Here's how the part is built. I have some questions about the finished solid (model axes, mm). A direction names the side the tool comes from. Give positions to 0.01 mm unless a question says otherwise; leave off trailing zeros. Write each loop counter-clockwise with the first axis right and the second up, starting at its lowest first coordinate (ties: lowest second). Pieces come first, ordered by that corner, then holes. Notation, with made-up numbers: (2, 65) -> (41, 65) arc R26 cw to (41, 86) -> close; hole circle Ø7 at (-10, 6.5). An arc over 180 degrees is marked (long way). Use one line per item in the form item = value.
Autodesk Inventor part; units mm, degrees
ref_plane "YZ Plane" through (0, 0, 0) normal (1, 0, 0) x (0, 1, 0)
ref_plane "XZ Plane" through (0, 0, 0) normal (0, 1, 0) x (-1, 0, 0)
ref_plane "XY Plane" through (0, 0, 0) normal (0, 0, 1) x (1, 0, 0)
sketch "Base" plane through (0, 0, 0) normal (0, 1, 0) x (-1, 0, 0)
  line L0 (92, 60.5) -> (-92, 60.5)
  line L1 (-92, 60.5) -> (-92, -60.5)
  line L2 (-92, -60.5) -> (92, -60.5)
  line L3 (92, -60.5) -> (92, 60.5)
  line L4 (92, 60.5) -> (-92, -60.5) construction
  line L5 (-92, 60.5) -> (92, -60.5) construction
  point P0 (0, 0)
  dimension "d0" = 184
  dimension "d1" = 121
extrude "Extrusão1" add sketch "Base" against normal blind 26
sketch "Esboço2" plane through (0, 0, 0) normal (0, 1, 0) x (1, 0, 0)
  line L0 (-90, -58.5) -> (90, -58.5)
  line L1 (90, -58.5) -> (90, 58.5)
  line L2 (90, 58.5) -> (-90, 58.5)
  line L3 (-90, 58.5) -> (-90, -58.5)
  line L4 (-90, -58.5) -> (90, 58.5) construction
  line L5 (90, -58.5) -> (-90, 58.5) construction
  point P0 (0, 0)
  dimension "d4" = 180
  dimension "d5" = 117
extrude "Extrusão2" cut sketch "Esboço2" against normal blind 22
sketch "Esboço3" plane through (0, -22, 0) normal (0, 1, 0) x (1, 0, 0)
  circle A0 centre (-85, -53.5) radius 2.5
  line L0 (-92, 60.5) -> (-92, -60.5)
  line L1 (-92, -60.5) -> (92, -60.5)
  circle A1 centre (-85, -53.5) radius 1.5
  line L2 (-90, -58.5) -> (-90, 58.5)
  line L3 (90, 58.5) -> (90, -58.5)
  circle A2 centre (-85, 53.5) radius 2.5
  circle A3 centre (-85, 53.5) radius 1.5
  line L4 (-90, 58.5) -> (90, 58.5)
  line L5 (90, -58.5) -> (-90, -58.5)
  circle A4 centre (85, 53.5) radius 1.5
  circle A5 centre (85, 53.5) radius 2.5
  line L6 (92, -60.5) -> (92, 60.5)
  line L7 (92, 60.5) -> (-92, 60.5)
  circle A6 centre (76.27, -28.99) radius 2.5
  circle A7 centre (76.27, -28.99) radius 1.5
  point P0 (0, 0)
  dimension "d8" = 5
  dimension "d9" = 7
  dimension "d10" = 7
  dimension "d11" = 3
  dimension "d12" = 7
  dimension "d13" = 7
  dimension "d14" = 5
  dimension "d15" = 31.51
  dimension "d16" = 15.73
  dimension "d17" = 3
extrude "Extrusão3" add sketch "Esboço3" along normal blind 4 contours A0 | A2 | A5 | A6
sketch "Esboço4" plane through (92, 0, -60.5) normal (0, 0, -1) x (-1, 0, 0)
  line L0 (92, 0) -> (64, 0)
  line L1 (64, 0) -> (64, -4)
  line L2 (64, -4) -> (92, -4)
  line L3 (92, -4) -> (92, 0)
  line L4 (92, 0) -> (64, -4) construction
  line L5 (64, 0) -> (92, -4) construction
  line L6 (184, 0) -> (184, -26)
  line L7 (0, 0) -> (184, 0)
  line L8 (184, -26) -> (0, -26)
  point P0 (92, 0)
  point P1 (78, -2)
  point P2 (64, -2)
  dimension "d20" = 120
  dimension "d21" = 28
  dimension "d22" = 0
  dimension "d24" = 4
extrude "Extrusão4" cut sketch "Esboço4" along normal blind 4 and the other way blind 2
properties part number "base_traseira_3DPrint"
Q1. I want a section at A-A, the plane z = -27. Write out the boundary of the cut face in (x, y).
Result set:
outline = (-92, -26) -> (92, -26) -> (92, 0) -> (90, 0) -> (90, -22) -> (-90, -22) -> (-90, 0) -> (-92, 0) -> close
Q2. If I drill on line 1 along Z through (x, y) = (-85, -19.6); line 2 along X through (y, z) = (-20.9, -53.5); line 3 along X through (y, z) = (-6.25, 45.5), over which ranges is the centre line in solid material (lowest first)? Write a range as from..to.
Result set:
line_1 = -60.5..-58.5, -56..-55, -52..-51, 51..52, 55..56, 58.5..60.5
line_2 = -92..-90, -87.5..-86.5, -83.5..-82.5, 82.5..83.5, 86.5..87.5, 90..92
line_3 = -92..-90, 90..92
Q3. I want a section at B-B, the plane y = -14.5. Write out the boundary of the cut face in (x, z), and give its area (3 significant figures).
Result set:
outline = (-92, -60.5) -> (92, -60.5) -> (92, 60.5) -> (-92, 60.5) -> close; hole (-90, -58.5) -> (90, -58.5) -> (90, 58.5) -> (-90, 58.5) -> close
area = 1,200 mm2
Q4. Will these pins go through, and if not, where does the flat tip stop? pin 1 Ø3.5 at (x, z) = (-85, -53.5) entering from +Y; pin 2 Ø12 at (x, z) = (-6.5, 23) entering from +Y; pin 3 Ø2 at (x, z) = (20, -59.5) entering from +Y.
Result set:
pin_1 = -18
pin_2 = -22
pin_3 = -4
Q5. If we mould it in two halves opening along Z, with no side actions, what happens to faces 1 (the face through (1, -26, 1)), 2 (the face through (1, -11, -58.5)), 3 (the face through (1, -13, -60.5))? For each: +Z half, -Z half, draft (parallel to the pull), parting line (faces both ways), or undercut.
Result set:
face_1 = draft
face_2 = undercut
face_3 = -Z half
Q6. I want a section at C-C, the plane x = -57. Write out the boundary of the cut face in (y, z).
Result set:
outline = (-26, -60.5) -> (0, -60.5) -> (0, -58.5) -> (-22, -58.5) -> (-22, 58.5) -> (0, 58.5) -> (0, 60.5) -> (-26, 60.5) -> close
Q7. Which directions (+Z, -Z, +X, -X, +Y, -Y) give clear straight access to the entire face, cutting with the end or side of a thin tool? Please do faces 4 (the face through (-87.5, -20, -53.4)), 5 (the face through (0, 0, 59)).
Result set:
face_4 = +Y
face_5 = +Z, -Z, +X, -X, +Y
